from build123d import *

# Parameters (mm, degrees)
F0_W     = 4.064
F0_H     = 3
F1_DEPTH = 15.24
F2_W     = 20
F2_H     = 25
F3_DEPTH = 40
F5_DEPTH = 25.001
F7_DEPTH = 20.001


# Not quite as in the source:
# - a pattern or mirror of a feature is missing from the dataset's text; its kind, count and spacing are read off the source's solid


with BuildPart() as f1:
    # F0 (on Front) → F1 (new body)
    with BuildSketch(Plane.XZ):
        Polygon((6.0325, 4.445), (-6.0325, 4.445), (-6.0325, 0), (-2.032, 0), (2.032, 0), (6.0325, 0), align=None)
        with Locations((0, -1.5)):
            Rectangle(F0_W, F0_H)
        Polygon((2.032, -3), (-2.032, -3), (-10, -3), (-10, -7), (10, -7), (10, -3), align=None)
    extrude(amount=-F1_DEPTH)

    # F2 (on face) → F3 (join)
    with BuildSketch(Plane.XZ):
        with Locations((0, 5.5)):
            Rectangle(F2_W, F2_H)
    extrude(amount=F3_DEPTH)

    # F4 (on face) → F5 (cut, through all)
    with BuildSketch(Plane.XY.offset(18)):
        Polygon((-3.305207938, -40), (-10, -7.6365470886), (-10, -40), align=None)
    f5 = extrude(amount=-F5_DEPTH, mode=Mode.SUBTRACT)

    # F5_copies: F5 across plane
    add(f5.mirror(Plane(origin=(0, 0, 0), x_dir=(0, 0, 1), z_dir=(1, 0, 0))), mode=Mode.SUBTRACT)

    # F6 (on face) → F7 (cut, through all)
    with BuildSketch(Plane.YZ.offset(10)):
        Polygon((-40, 18), (-40, 4), (-7.6365470886, 18), align=None)
    extrude(amount=-F7_DEPTH, mode=Mode.SUBTRACT)


solid = f1.part
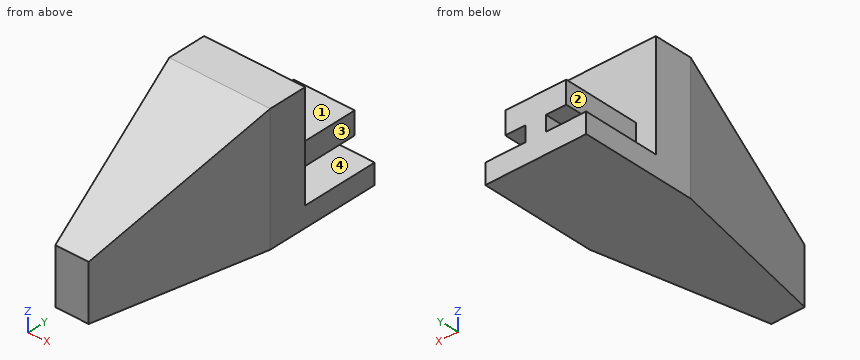
Source: CAD feature listing. Evaluate the final solid. Frame: model axes, mm. Face numbers are marked on the shaded views. A direction names the side the tool comes from. Coordinates: 2 decimals unless noted, no trailing zeros. Loops run counter-clockwise (first coordinate to the right, second up) from the corner with the lowest first, then second, coordinate; pieces in that order, holes last. Notation, with made-up numbers: (36, 56) -> (84, 56) arc R23 ccw to (84, 83) -> close; hole circle Ø4 at (56.5, -25.75). An arc over 180 degrees is marked (long way). Answer in a Markdown table with one row per item. Add a question column.
Q1. Section B-B on y = 1. Return the cut outline in (x, z) (1 decimal), and give its area (3 significant figures).
Q2. Section D-D on z = -5.5. Return the cut outline in (x, y), and give its area (3 significant figures).
Q3. Section C-C on x = -4.25. Return the cut outline in (y, z) (3 decimals).
Q4. Ray query, line 1 along Z through (x, y) = (5.25, 3.5) (3 decimals); line 2 along Z through (x, y) = (-7.5, -14); line 3 along X through (y, z) = (5.5, -2.5). Return the intervals inside material, ascending.
Q5. Reachability of the marked faces 1, 2, 3 and 4 from +Z, -Z, +X, -X, +Y, -Y: full face, straight path, thin tool, end or side. Return the list, or none.
Q6. Contact query for flat-ended pins moving along their axis: pin 1 Ø10 at (x, y) = (-7.5, -13.5) entering from +Z; pin 2 Ø3 at (y, z) = (2.5, 4) entering from -X; pin 3 Ø6 at (x, y) = (-2, 11.5) entering from +Z (3 decimals). Output: stop coordinate, or through.
Q7. Section A-A on z = -1.5. Return the cut outline in (x, y).
Computed values:
| question | item | result |
|---|---|---|
| 1 | outline | (-10, -7) -> (10, -7) -> (10, -3) -> (2, -3) -> (2, 0) -> (6, 0) -> (6, 4.4) -> (-6, 4.4) -> (-6, 0) -> (-2, 0) -> (-2, -3) -> (-10, -3) -> close |
| 1 | area | 146 mm^2 |
| 2 | outline | (-10, -7.64) -> (-3.31, -40) -> (3.31, -40) -> (10, -7.64) -> (10, 15.24) -> (-10, 15.24) -> close |
| 2 | area | 888 mm^2 |
| 3 | outline | (-35.433, -7) -> (15.24, -7) -> (15.24, -3) -> (0, -3) -> (0, 0) -> (15.24, 0) -> (15.24, 4.445) -> (0, 4.445) -> (0, 18) -> (-7.637, 18) -> (-35.433, 5.976) -> close |
| 4 | line 1 | z = -7 to -3, 0 to 4.445 |
| 4 | line 2 | z = -7 to 15.25 |
| 4 | line 3 | x = -2.03 to 2.03 |
| 5 | face 1 | +Z, +X, -X, +Y |
| 5 | face 2 | +Z, -X, +Y |
| 5 | face 3 | +Z, +X, +Y |
| 5 | face 4 | +X, +Y |
| 6 | pin 1 | stops at z = 17.63 |
| 6 | pin 2 | stops at x = -6.03 |
| 6 | pin 3 | stops at z = 4.445 |
| 7 | outline | (-10, -7.64) -> (-3.31, -40) -> (3.31, -40) -> (10, -7.64) -> (10, 0) -> (2.03, 0) -> (2.03, 15.24) -> (-2.03, 15.24) -> (-2.03, 0) -> (-10, 0) -> close |
